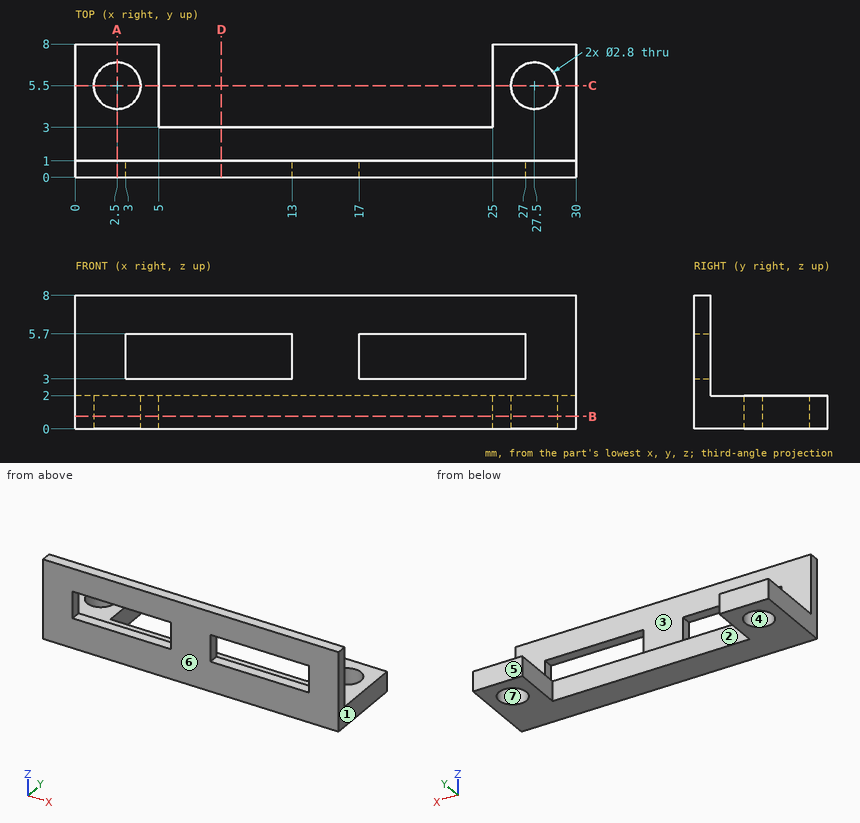
Drawing for the job (mm, zero at the part's lowest x, y, z). A direction names the side the tool comes from. Round coordinates to 2 decimals unless told otherwise and drop trailing zeros. Write each loop counter-clockwise with the first axis right and the second up, starting at its lowest first coordinate (ties: lowest second). Pieces come first, ordered by that corner, then holes. Notation, with made-up numbers: (-12.5, 20.25) - (1.5, 20.25) arc R16 ccw to (1.5, 25.25) - close; hole circle Ø6 at (-37, 17.25). An arc over 180 degrees is marked (long way). Write item = value, one per line. Start each with the question number.
Q1. Band-saw the part on D-D (x = 8.75). Give the cut face in (y, z), then the cut area to 3 significant figures.
Q2. Band-saw the part on B-B (z = 0.75). Give the cut face in (x, y), then the cut area to 3 significant figures.
Q3. Band-saw the part on A-A (x = 2.5). Give the cut face in (y, z), then the cut area to 3 significant figures.
Q4. Band-saw the part on C-C (y = 5.5). Give the cut face in (x, z).
Q5. Probe L1, parallel to X at y = 5.5, z = 0.7; L2, parallel to X at y = 0.5, z = 4.25; L3, parallel to Z at x = 6, y = 0.5. List the from-to ranges inside material, lowest first. Write a range as from..to.
Q6. Mould opens along Y. For the marked faces 4, 5, 6 and 7 say: pulls with the +Y half, pulls with the -Y half, needs draft (parallel to the pull), parting line crosses it, or undercut.
Q7. Which spindle directions (+Z, -Z, +X, -X, +Y, -Y) get a long thin tool onto all of the face, cutting with end or side? Do the marked faces 1, 2 and 3. Say none if no direction does.
Q8. Drop flat-ended pins along their axis: pin 1 (1.8 mm diameter, centred on x = 18.5, z = 6, fed in from +Y); pin 2 (1.6 mm diameter, centred on x = 12.5, z = 1, fed in from +Y); pin 3 (1.5 mm diameter, centred on x = 26.5, y = 2, fed in from +Z). Give the stop position or say it passes through.
Answers below:
q1.outline = (0, 0) - (3, 0) - (3, 2) - (1, 2) - (1, 3) - (0, 3) - close; (0, 5.7) - (1, 5.7) - (1, 8) - (0, 8) - close
q1.area = 9.30 mm2
q2.outline = (0, 0) - (30, 0) - (30, 8) - (25, 8) - (25, 3) - (5, 3) - (5, 8) - (0, 8) - close; hole circle Ø2.8 at (2.5, 5.5); hole circle Ø2.8 at (27.5, 5.5)
q2.area = 128 mm2
q3.outline = (0, 0) - (4.1, 0) - (4.1, 2) - (1, 2) - (1, 8) - (0, 8) - close; (6.9, 0) - (8, 0) - (8, 2) - (6.9, 2) - close
q3.area = 16.4 mm2
q4.outline = (0, 0) - (1.1, 0) - (1.1, 2) - (0, 2) - close; (3.9, 0) - (5, 0) - (5, 2) - (3.9, 2) - close; (25, 0) - (26.1, 0) - (26.1, 2) - (25, 2) - close; (28.9, 0) - (30, 0) - (30, 2) - (28.9, 2) - close
q5.L1 = 0..1.1, 3.9..5, 25..26.1, 28.9..30
q5.L2 = 0..3, 13..17, 27..30
q5.L3 = 0..3, 5.7..8
q6.face_4 = undercut
q6.face_5 = pulls with the +Y half
q6.face_6 = pulls with the -Y half
q6.face_7 = undercut
q7.face_1 = +Z, -Z, +X, +Y, -Y
q7.face_2 = +Z, -Z, +Y
q7.face_3 = +Z, +X, -X, +Y
q8.pin_1 = 1
q8.pin_2 = 3
q8.pin_3 = 2
